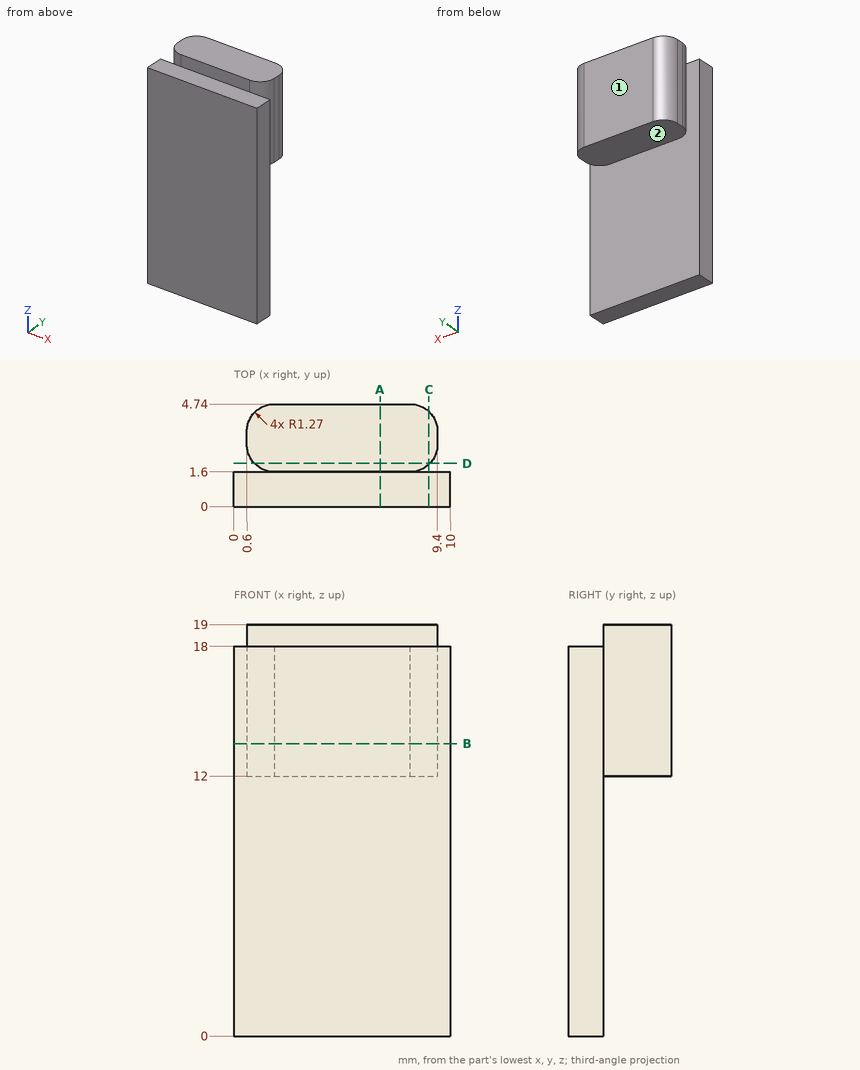
Design review of the part shown in the three views and the two pictorial views. Dimensions are in mm from the part's minimum x, y and z. A direction names the side the tool comes from. Round coordinates to 2 decimals unless told otherwise and drop trailing zeros. Write each loop counter-clockwise with the first axis right and the second up, starting at its lowest first coordinate (ties: lowest second). Pieces come first, ordered by that corner, then holes. Notation, with made-up numbers: M 66,14 L 96,14 A9 ccw 96,29 Z; hole C 49,73 d7. An arc over 180 degrees is marked long. Use a Markdown table: item, result. Add a question column.
Q1. To check wall thickness, follow line 1 (Z direction, x = 6.5, y = 1.4); line 2 (Z direction, x = 5, y = 3.55); line 3 (X direction, y = 3.4, z = 15.5). State the ranges of each line that lie inside material, in increasing order.
Q2. Machinability: for the marked faces 1 and 2, which of the approach directions +Z, -Z, +X, -X, +Y, -Y give a long, thin tool a straight path to every point of the face, cutting with its end or side? Answer none if there is none.
Q3. Insertion check: pin 1 (1.5 mm diameter, centred on x = 6.5, y = 3, fed in from -Z); pin 2 (1.3 mm diameter, centred on x = 7.5, y = 0.5, fed in from +Z); pin 3 (0.5 mm diameter, centred on y = 3.5, z = 16, fed in from -X). Each pin has a flat end and moves straight along its axis. Give the tip position at first contact, or say it passes through.
Q4. We need section C-C, the plane x = 9. State the section outline as (y, z) points, plus the area to 3 significant figures.
Q5. We need section A-A, the plane x = 6.75. State the section outline as (y, z) points.
Q6. We need section D-D, the plane y = 2. State the section outline as (x, z) points, plus the area to 3 significant figures.
Q7. We need section B-B, the plane z = 13.5. State the section outline as (x, y) points.
Findings below:
| question | item | result |
|---|---|---|
| 1 | line 1 | z = 0 to 18 |
| 1 | line 2 | z = 12 to 19 |
| 1 | line 3 | x = 0.6 to 9.4 |
| 2 | face 1 | +Z, -Z, +X, -X, +Y |
| 2 | face 2 | -Z, +X, -X, +Y |
| 3 | pin 1 | stops at z = 12 |
| 3 | pin 2 | stops at z = 18 |
| 3 | pin 3 | stops at x = 0.6 |
| 4 | outline | M 0,0 L 1.6,0 L 1.6,18 L 0,18 Z; M 1.94,12 L 4.4,12 L 4.4,19 L 1.94,19 Z |
| 4 | area | 46.0 mm² |
| 5 | outline | M 0,0 L 1.6,0 L 1.6,12 L 4.74,12 L 4.74,19 L 1.6,19 L 1.6,18 L 0,18 Z |
| 6 | outline | M 0.94,12 L 9.06,12 L 9.06,19 L 0.94,19 Z |
| 6 | area | 56.8 mm² |
| 7 | outline | M 0,0 L 10,0 L 10,1.6 L 8.13,1.6 A1.27 ccw 9.4,2.87 L 9.4,3.47 A1.27 ccw 8.13,4.74 L 1.87,4.74 A1.27 ccw 0.6,3.47 L 0.6,2.87 A1.27 ccw 1.87,1.6 L 0,1.6 Z |
